Source: CAD feature listing. Evaluate the final solid. Frame: model axes, mm. Give positions to 0.01 mm unless a question says otherwise; leave off trailing zeros. Order: outer loops, then holes, each group sorted by start corner. A loop starts at its lowest first (then second) coordinate and runs counter-clockwise, first axis right, second up.
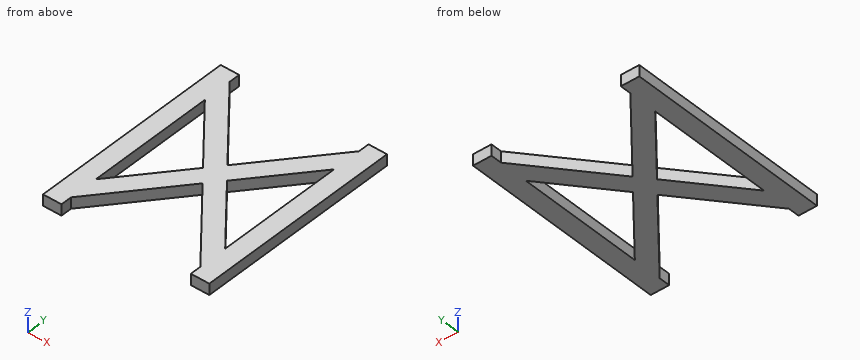
from build123d import *

# Parameters (mm, degrees)
BOSS_EXTRUDE1_DEPTH = 3


with BuildPart() as part:
    # Sketch1 → Boss-Extrude1 (new body)
    with BuildSketch(Plane.XY):
        Polygon((0, 56), (0, 28), (5, 28), (5, 45.17097131), (5, 53), (5, 56), align=None)
        Polygon((5, 53), (5, 45.17097131), (19.251130035, 28), (22.5, 31.914514345), align=None)
        Polygon((0, 28), (0, 0), (5, 0), (5, 3), (5, 10.82902869), (5, 28), align=None)
        Polygon((5, 10.82902869), (5, 3), (22.5, 24.085485655), (19.251130035, 28), align=None)
        Polygon((25.748869965, 28), (19.251130035, 28), (22.5, 24.085485655), align=None)
        Polygon((22.5, 31.914514345), (25.748869965, 28), (40, 45.17097131), (40, 53), align=None)
        Polygon((40, 45.17097131), (40, 28), (45, 28), (45, 56), (40, 56), (40, 53), align=None)
        Polygon((40, 10.82902869), (40, 3), (40, 0), (45, 0), (45, 28), (40, 28), align=None)
        Polygon((25.748869965, 28), (22.5, 24.085485655), (40, 3), (40, 10.82902869), align=None)
        Polygon((22.5, 31.914514345), (19.251130035, 28), (25.748869965, 28), align=None)
    extrude(amount=BOSS_EXTRUDE1_DEPTH)


solid = part.part
1) Section query D-D on y = 51.5. Output: boundary loops of the cut face in (x, z).
Checks:
outline: (0, 0) - (6.24, 0) - (6.24, 3) - (0, 3) - close; (38.76, 0) - (45, 0) - (45, 3) - (38.76, 3) - close
2) Section query C-C on y = 33. Output: boundary loops of the cut face in (x, z).
Checks:
outline: (0, 0) - (5, 0) - (5, 3) - (0, 3) - close; (15.1, 0) - (21.6, 0) - (21.6, 3) - (15.1, 3) - close; (23.4, 0) - (29.9, 0) - (29.9, 3) - (23.4, 3) - close; (40, 0) - (45, 0) - (45, 3) - (40, 3) - close
3) Ray query, L1, parallel to X at y = 29, z = 0.35; L2, parallel to X at y = 28.5, z = 2.4; L3, parallel to X at y = 20, z = 1.15. Return the intervals inside material, ascending.
Checks:
L1: x = 0 to 5, 18.42 to 26.58, 40 to 45
L2: x = 0 to 5, 18.84 to 26.16, 40 to 45
L3: x = 0 to 5, 12.61 to 19.11, 25.89 to 32.39, 40 to 45
4) First-contact query: pin 1 Ø1.5 at (x, z) = (27, 2.5) entering from -Y. Flat tip, straight axial feed; report the tip coordinate or a pass-through.
Checks:
pin 1: stops at y = 17.76
5) Section query A-A on z = 2.55. Output: boundary loops of the cut face in (x, y), and give its area (3 significant figures).
Checks:
outline: (0, 0) - (5, 0) - (5, 3) - (22.5, 24.09) - (40, 3) - (40, 0) - (45, 0) - (45, 56) - (40, 56) - (40, 53) - (22.5, 31.91) - (5, 53) - (5, 56) - (0, 56) - close; hole (5, 10.83) - (19.25, 28) - (5, 45.17) - close; hole (25.75, 28) - (40, 10.83) - (40, 45.17) - close
area: 1,080 mm2
6) Section query B-B on x = 27. Output: boundary loops of the cut face in (y, z).
Checks:
outline: (18.66, 0) - (26.49, 0) - (26.49, 3) - (18.66, 3) - close; (29.51, 0) - (37.34, 0) - (37.34, 3) - (29.51, 3) - close
